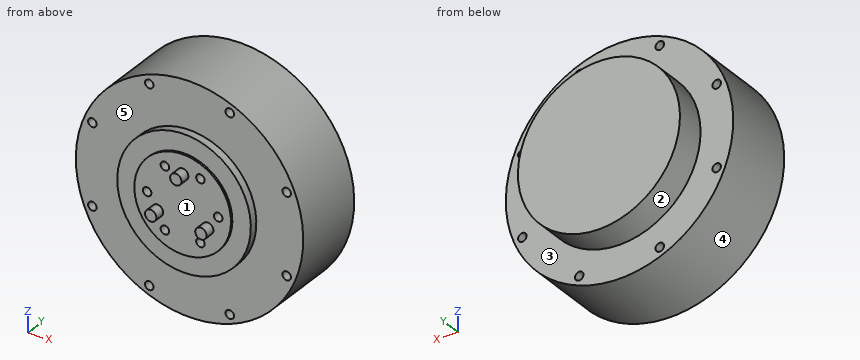
```python
from build123d import *

# Parameters (mm, degrees)
EXTRUDE_1_DEPTH      = 13
EXTRUDE_1_DEPTH_BACK = 13
SKETCH_1_R           = 40
SKETCH_2_R           = 28.5
EXTRUDE_2_DEPTH      = 10.5
SKETCH_3_R           = 23.5
EXTRUDE_3_DEPTH      = 2.8
SKETCH_4_R           = 17
EXTRUDE_4_DEPTH      = 0.7
SKETCH_5_R           = 1.5
CUT_EXTRUDE_1_DEPTH  = 5
CUT_EXTRUDE_START    = 5
SKETCH_6_R           = 1.5
CUT_EXTRUDE_3_DEPTH  = 5
SKETCH_7_R           = 1.5
CUT_EXTRUDE_4_DEPTH  = 5
SKETCH_8_R           = 2
EXTRUDE_5_DEPTH      = 3.5


with BuildPart() as part:
    # Sketch 1 → Extrude 1 (new, two sides: drawn at the far end of the back side and taken through both)
    with BuildSketch(Plane(origin=(0, 0, 0), x_dir=(1, 0, 0), z_dir=(0, 1, 0)).offset(-EXTRUDE_1_DEPTH_BACK)):
        with Locations(Location((0, 0, 0), (0, 0, 270))):
            Circle(SKETCH_1_R)
    extrude(amount=EXTRUDE_1_DEPTH + EXTRUDE_1_DEPTH_BACK)

    # Sketch 2 → Extrude 2 (add)
    with BuildSketch(Plane(origin=(0, 13, 0), x_dir=(1, 0, 0), z_dir=(0, 1, 0))):
        with Locations(Location((0, 0, 0), (0, 0, 90))):
            Circle(SKETCH_2_R)
    extrude(amount=EXTRUDE_2_DEPTH)

    # Sketch 3 → Extrude 3 (add)
    with BuildSketch(Plane.XZ.offset(13)):
        with Locations(Location((0, 0, 0), (0, 0, 270))):
            Circle(SKETCH_3_R)
    extrude(amount=EXTRUDE_3_DEPTH)

    # Sketch 4 → Extrude 4 (add)
    with BuildSketch(Plane.XZ.offset(15.8)):
        with Locations(Location((0, 0, 0), (0, 0, 270))):
            Circle(SKETCH_4_R)
    extrude(amount=EXTRUDE_4_DEPTH)

    # Sketch 5 → Cut-Extrude 1 (cut)
    with BuildSketch(Plane(origin=(0, 13, 0), x_dir=(1, 0, 0), z_dir=(0, 1, 0))):
        with Locations(Location((14.159286998, 34.183542703, 0), (0, 0, 270))):
            Circle(SKETCH_5_R)
        with Locations(Location((34.183542703, 14.159286998, 0), (0, 0, 90))):
            Circle(SKETCH_5_R)
        with Locations(Location((34.183542703, -14.159286998, 0), (0, 0, 270))):
            Circle(SKETCH_5_R)
        with Locations(Location((14.159286998, -34.183542703, 0), (0, 0, 90))):
            Circle(SKETCH_5_R)
        with Locations(Location((-14.159286998, -34.183542703, 0), (0, 0, 270))):
            Circle(SKETCH_5_R)
        with Locations(Location((-34.183542703, -14.159286998, 0), (0, 0, 90))):
            Circle(SKETCH_5_R)
        with Locations(Location((-34.183542703, 14.159286998, 0), (0, 0, 270))):
            Circle(SKETCH_5_R)
        with Locations(Location((-14.159286998, 34.183542703, 0), (0, 0, 90))):
            Circle(SKETCH_5_R)
    extrude(amount=-CUT_EXTRUDE_1_DEPTH, mode=Mode.SUBTRACT)

    # Sketch 6 → Cut-Extrude 3 (cut)
    with BuildSketch(Plane(origin=(0, -13, -13), x_dir=(1, 0, 0), z_dir=(0, 1, 0)).offset(CUT_EXTRUDE_START)):
        with Locations(Location((14.159286998, 21.183542703, 0), (0, 0, 270))):
            Circle(SKETCH_6_R)
        with Locations(Location((34.183542703, 1.159286998, 0), (0, 0, 90))):
            Circle(SKETCH_6_R)
        with Locations(Location((34.183542703, -27.159286998, 0), (0, 0, 270))):
            Circle(SKETCH_6_R)
        with Locations(Location((14.159286998, -47.183542703, 0), (0, 0, 90))):
            Circle(SKETCH_6_R)
        with Locations(Location((-14.159286998, -47.183542703, 0), (0, 0, 270))):
            Circle(SKETCH_6_R)
        with Locations(Location((-34.183542703, -27.159286998, 0), (0, 0, 90))):
            Circle(SKETCH_6_R)
        with Locations(Location((-34.183542703, 1.159286998, 0), (0, 0, 270))):
            Circle(SKETCH_6_R)
        with Locations(Location((-14.159286998, 21.183542703, 0), (0, 0, 90))):
            Circle(SKETCH_6_R)
    extrude(amount=-CUT_EXTRUDE_3_DEPTH, mode=Mode.SUBTRACT)

    # Sketch 7 → Cut-Extrude 4 (cut)
    with BuildSketch(Plane.XZ.offset(16.5)):
        with Locations(Location((-12.5, 0, 0), (0, 0, 270))):
            Circle(SKETCH_7_R)
        with Locations(Location((-6.25, 10.825317547, 0), (0, 0, 270))):
            Circle(SKETCH_7_R)
        with Locations(Location((-6.25, -10.825317547, 0), (0, 0, 90))):
            Circle(SKETCH_7_R)
        with Locations(Location((6.25, -10.825317547, 0), (0, 0, 270))):
            Circle(SKETCH_7_R)
        with Locations(Location((12.5, 0, 0), (0, 0, 90))):
            Circle(SKETCH_7_R)
        with Locations(Location((6.25, 10.825317547, 0), (0, 0, 90))):
            Circle(SKETCH_7_R)
    extrude(amount=-CUT_EXTRUDE_4_DEPTH, mode=Mode.SUBTRACT)

    # Sketch 8 → Extrude 5 (add)
    with BuildSketch(Plane.XZ.offset(16.5)):
        with Locations(Location((0, 10.2, 0), (0, 0, 270))):
            Circle(SKETCH_8_R)
        with Locations(Location((-8.833459119, -5.1, 0), (0, 0, 270))):
            Circle(SKETCH_8_R)
        with Locations(Location((8.833459119, -5.1, 0), (0, 0, 90))):
            Circle(SKETCH_8_R)
    extrude(amount=EXTRUDE_5_DEPTH)


solid = part.part
```
Geometry: final body of the model. Coordinates: model frame, mm. Face numbers are marked on the shaded views. A direction names the side the tool comes from. Round coordinates to 2 decimals unless told otherwise and drop trailing zeros. Write each loop counter-clockwise with the first axis right and the second up, starting at its lowest first coordinate (ties: lowest second). Pieces come first, ordered by that corner, then holes. Notation, with made-up numbers: (89.5, 67.5) -> (110.5, 67.5) arc R13 cw to (110.5, 72.5) -> close; hole circle Ø8 at (33.5, 22). An arc over 180 degrees is marked (long way). Return JSON: item names as keys, results as strings.
Q1. Set-up query: the marked faces 3, 4 and 5. Return all of +Z, -Z, +X, -X, +Y, -Y with unobstructed straight access to the full face (end or side cutting, diameter ignored); none if empty.
From the geometry:
{"face 3": "+Y", "face 4": "+Y, -Y", "face 5": "-Y"}
Q2. Section A-A on z = 0. Return the cut outline in (x, y).
From the geometry:
{"outline": "(-40, -13) -> (-23.5, -13) -> (-23.5, -15.8) -> (-17, -15.8) -> (-17, -16.5) -> (-14, -16.5) -> (-14, -11.5) -> (-11, -11.5) -> (-11, -16.5) -> (11, -16.5) -> (11, -11.5) -> (14, -11.5) -> (14, -16.5) -> (17, -16.5) -> (17, -15.8) -> (23.5, -15.8) -> (23.5, -13) -> (40, -13) -> (40, 13) -> (28.5, 13) -> (28.5, 23.5) -> (-28.5, 23.5) -> (-28.5, 13) -> (-40, 13) -> close"}
Q3. Section D-D on x = 27. Return the cut outline in (y, z).
From the geometry:
{"outline": "(-13, -29.51) -> (13, -29.51) -> (13, -9.12) -> (23.5, -9.12) -> (23.5, 9.12) -> (13, 9.12) -> (13, 29.51) -> (-13, 29.51) -> close"}
Q4. Ray query, line 1 (Z direction, x = -6, y = -15); line 2 (Y direction, x = 19.5, z = -30); line 3 (Y direction, x = 16, z = -21). Return the intervals inside material, ascending.
From the geometry:
{"line 1": "-22.72 to -12.3, -9.35 to 9.35, 12.3 to 22.72", "line 2": "-13 to 13", "line 3": "-13 to 23.5"}
Q5. Section C-C on y = -5. Return the cut outline in (x, z).
From the geometry:
{"outline": "circle Ø80 at (0, 0)"}
Q6. Mould query, pull axis Z, two halves, no side actions, for the marked faces 1 and 2. Classes: +Z half, -Z half, draft (parallel to the pull), parting line (faces both ways), or undercut.
From the geometry:
{"face 1": "draft", "face 2": "parting line"}
Q7. Section B-B on x = 0. Return the cut outline in (y, z).
From the geometry:
{"outline": "(-20, 8.2) -> (-16.5, 8.2) -> (-16.5, -17) -> (-15.8, -17) -> (-15.8, -23.5) -> (-13, -23.5) -> (-13, -40) -> (13, -40) -> (13, -28.5) -> (23.5, -28.5) -> (23.5, 28.5) -> (13, 28.5) -> (13, 40) -> (-13, 40) -> (-13, 23.5) -> (-15.8, 23.5) -> (-15.8, 17) -> (-16.5, 17) -> (-16.5, 12.2) -> (-20, 12.2) -> close"}
Q8. First-contact query: pin 1 Ø4 at (x, y) = (29, -0.5) entering from +Z; pin 2 Ø3.5 at (x, z) = (13.5, 34) entering from -Y; pin 3 Ø0.9 at (x, z) = (-14, -33.5) entering from +Y; pin 4 Ø1.5 at (x, y) = (-29.5, 18.5) entering from -Z. Flat tips, straight axial feed; report the tip coordinate or a pass-through.
From the geometry:
{"pin 1": "z = 29.51", "pin 2": "y = -13", "pin 3": "y = 8", "pin 4": "through"}
